Verification items for the finished model (mm, model axes). A direction names the side the tool comes from. Give positions to 0.01 mm unless a question says otherwise; leave off trailing zeros. Order: outer loops, then holes, each group sorted by start corner. A loop starts at its lowest first (then second) coordinate and runs counter-clockwise, first axis right, second up. Notation, with made-up numbers: (56.25, -37) -> (63.25, -37) arc R16 ccw to (63.25, -8) -> close; hole circle Ø3 at (78, 54). An arc over 180 degrees is marked (long way). Return JSON: item names as keys, results as strings. Group by question number.
(1) Cross-section at C-C on x = 9. Enter the section's corners in (y, z).
(2) Cross-section at D-D on y = -3. Enter the section's corners in (x, z).
(3) Depth check by flat-ended pin: pin 1 Ø3 at (y, z) = (-4, -3) entering from -X; pin 2 Ø4 at (x, y) = (0, -5.5) entering from -Z; pin 3 Ø1.5 at (x, z) = (-8.5, -4) entering from -Y; pin 4 Ø5 at (x, y) = (9, -10) entering from +Z. Enter the tip coordinate at first touch or a pass-through.
(4) Thickness scan on line 1 along X through (y, z) = (-4.5, 2.5); line 2 along Y through (x, z) = (-9, -4); line 3 along X through (y, z) = (-12.5, 5.5). Record the ranges inside material, lowest first.
(5) Cross-section at B-B on y = -8.75. Enter the section's corners in (x, z).
(6) Cross-section at A-A on z = 0. Enter the section's corners in (x, y).
(7) Tool access check on faces 4 (the face through (-8, -7.4, -1.5)), 5 (the face through (11, -10, -2)), 6 (the face through (-6, -8, -1)), 7 (the face through (0, -8, 6.7)), 8 (the face through (-8, -6, -3)). Record the directions out of +Z, -Z, +X, -X, +Y, -Y that give a thin tool (end or side, any length) a straight path to the whole face; none if there is none.
(8) Release check for a two-part mould opening along Y. For faces 1 (the face through (-7.5, -8, 1)), 2 (the face through (8, -13.9, -3)), 3 (the face through (-7.474, -9.519, -3.472)) record: pulls with the +Y half, pulls with the -Y half, needs draft (parallel to the pull), parting line crosses it, or undercut.
from build123d import *

# Parameters (mm, degrees)
PAD012_DEPTH    = 11.5
FILLET001_R     = 1
FILLET002_R     = 2
SKETCH019_W     = 5.8
SKETCH019_H     = 7.9
PAD013_DEPTH    = 3
CHAMFER_SIZE    = 1
FILLET003_R     = 3.9
SKETCH020_R     = 1.6
POCKET006_DEPTH = 4


with BuildPart() as part:
    # Sketch018 (on DatumPlane) → Pad012 (new body)
    with BuildSketch(Plane.XZ.offset(2.5)):
        Polygon((-7.5, -5), (-7.5, 6.7), (7.5, 6.7), (7.5, -5), (6, -5), (6, 5), (-6, 5), (-6, -5), align=None)
    extrude(amount=PAD012_DEPTH)

    # Fillet001
    fillet001_edges = [part.edges().sort_by_distance(p)[0] for p in [
        (-7.5, -8.25, 6.7),
        (7.5, -8.25, 6.7),
    ]]
    fillet(fillet001_edges, radius=FILLET001_R)

    # Fillet002
    fillet002_edges = [part.edges().sort_by_distance(p)[0] for p in [
        (6, -8.25, 5),
        (-6, -8.25, 5),
    ]]
    fillet(fillet002_edges, radius=FILLET002_R)

    # Sketch019 (on DatumPlane) → Pad013 (join)
    with BuildSketch(Plane.XY.offset(-5)):
        with Locations((10.4, -9.95)):
            Rectangle(SKETCH019_W, SKETCH019_H)
        with Locations((-10.4, -9.95)):
            Rectangle(SKETCH019_W, SKETCH019_H)
    extrude(amount=PAD013_DEPTH)

    # Chamfer
    chamfer_edges = [part.edges().sort_by_distance(p)[0] for p in [
        (7.5, -9.95, -2),
        (-7.5, -9.95, -2),
    ]]
    chamfer(chamfer_edges, length=CHAMFER_SIZE)

    # Fillet003
    fillet003_edges = [part.edges().sort_by_distance(p)[0] for p in [
        (13.3, -6, -3.5),
        (13.3, -13.9, -3.5),
        (-13.3, -13.9, -3.5),
        (-13.3, -6, -3.5),
    ]]
    fillet(fillet003_edges, radius=FILLET003_R)

    # Sketch020 (on DatumPlane) → Pocket006 (cut)
    with BuildSketch(Plane.XY.offset(-5)):
        with Locations((-9, -10)):
            Circle(SKETCH020_R)
        with Locations((9, -10)):
            Circle(SKETCH020_R)
    extrude(amount=POCKET006_DEPTH, mode=Mode.SUBTRACT)


solid = part.part
Verdict:
{
 "1": {"outline": "(-13.9, -5) -> (-11.6, -5) -> (-11.6, -2) -> (-13.9, -2) -> close; (-8.4, -5) -> (-6, -5) -> (-6, -2) -> (-8.4, -2) -> close"},
 "2": {"outline": "(-7.5, -5) -> (-6, -5) -> (-6, 3) arc R2 cw to (-4, 5) -> (4, 5) arc R2 cw to (6, 3) -> (6, -5) -> (7.5, -5) -> (7.5, 5.7) arc R1 ccw to (6.5, 6.7) -> (-6.5, 6.7) arc R1 ccw to (-7.5, 5.7) -> close"},
 "3": {"pin 1": "x = -7.5", "pin 2": "z = 5", "pin 3": "y = -13.9", "pin 4": "z = 6.7"},
 "4": {"line 1": "-7.5 to -6, 6 to 7.5", "line 2": "-13.9 to -11.6, -8.4 to -6", "line 3": "-7.5 to 7.5"},
 "5": {"outline": "(-13.13, -5) -> (-10, -5) -> (-10, -2) -> (-13.13, -2) -> close; (-8, -5) -> (-6, -5) -> (-6, 3) arc R2 cw to (-4, 5) -> (4, 5) arc R2 cw to (6, 3) -> (6, -5) -> (8, -5) -> (8, -1.5) -> (7.5, -1) -> (7.5, 5.7) arc R1 ccw to (6.5, 6.7) -> (-6.5, 6.7) arc R1 ccw to (-7.5, 5.7) -> (-7.5, -1) -> (-8, -1.5) -> close; (10, -5) -> (13.13, -5) -> (13.13, -2) -> (10, -2) -> close"},
 "6": {"outline": "(-7.5, -14) -> (-6, -14) -> (-6, -2.5) -> (-7.5, -2.5) -> close; (6, -14) -> (7.5, -14) -> (7.5, -2.5) -> (6, -2.5) -> close"},
 "7": {"face 4": "+Z, -X, +Y, -Y", "face 5": "+Z, +X, +Y, -Y", "face 6": "-Z, +Y, -Y", "face 7": "+Z, +X, -X, +Y, -Y", "face 8": "+Z, -Z, -X, +Y"},
 "8": {"face 1": "needs draft", "face 2": "pulls with the -Y half", "face 3": "undercut"}
}
